Source: CAD feature listing. Evaluate the final solid. Frame: model axes, mm. Coordinates: 2 decimals unless noted, no trailing zeros. Loops run counter-clockwise (first coordinate to the right, second up) from the corner with the lowest first, then second, coordinate; pieces in that order, holes last.
Item 1: Section query C-C, the plane x = 36. Return the cut outline in (y, z).
Item 2: Section query B-B, the plane x = 30. Return the cut outline in (y, z).
Item 3: Pin query (flat end, axial travel): pin 1 Ø1.1 at (y, z) = (-6.5, 0.5) entering from -X (3 decimals); pin 2 Ø1.2 at (x, z) = (11, 0) entering from -Y; pin 3 Ø0.9 at (x, z) = (-12, 0) entering from +Y. Return the tip coordinate at first contact, or that it passes through.
Item 4: Section query A-A, the plane y = 0. Return the cut outline in (x, z) (3 decimals), then the cut area to 3 significant figures.
Item 5: Section query D-D, the plane x = 18. Return the cut outline in (y, z), then the cut area to 3 significant figures.
Item 6: Line query: probe 1 along Y at (x, z) = (30, -0.65); probe 2 along X at (y, z) = (0.5, -0.7) (3 decimals); probe 3 along X at (y, z) = (9, -1.1). Output: solid intervals per line, ascending.
```python
from build123d import *

# Parameters (mm, degrees)
EXTRUDE_1_DEPTH     = 1.25
SKETCH_2_R          = 0.6
CUT_EXTRUDE_1_DEPTH = 3.5
FILLET_1_R          = 0.5
SKETCH_3_R          = 10.5
CUT_EXTRUDE_2_DEPTH = 3.5
CHAMFER_1_SIZE      = 5
CHAMFER_2_SIZE      = 15
CHAMFER_3_SIZE      = 3
CUT_EXTRUDE_4_DEPTH = 3.5
SKETCH_6_R          = 1.55
CUT_EXTRUDE_5_DEPTH = 3.5


with BuildPart() as part:
    # 草图1 → 凸台-拉伸1 (new body, symmetric)
    with BuildSketch(Plane.XY):
        Polygon((-13, 20), (-13, 7.475), (-10.025, 7.475), (-10.025, 4), (-13.025, 4), (-13.025, -4), (-10.025, -4), (-10.025, -7.475), (-13, -7.475), (-13, -30), (42.5, -30), (42.5, 20), align=None)
        Polygon((10.025, 7.475), (10.025, 4), (13.025, 4), (13.025, -4), (10.025, -4), (10.025, -7.475), (16.125, -7.475), (16.125, 7.475), align=None, mode=Mode.SUBTRACT)
    extrude(amount=EXTRUDE_1_DEPTH, both=True)

    # 草图2 → 切除-拉伸1 (cut, through all)
    with BuildSketch(Plane.XY.offset(1.25)):
        with Locations((10.625, 7.475)):
            Circle(SKETCH_2_R)
        with Locations((16.125, 6.875)):
            Circle(SKETCH_2_R)
        with Locations((10.025, 4.6)):
            Circle(SKETCH_2_R)
        with Locations((10.025, -4.6)):
            Circle(SKETCH_2_R)
        with Locations((10.625, -7.475)):
            Circle(SKETCH_2_R)
        with Locations((16.125, -6.875)):
            Circle(SKETCH_2_R)
        with Locations((-10.025, -4.6)):
            Circle(SKETCH_2_R)
        with Locations((-10.625, -7.475)):
            Circle(SKETCH_2_R)
        with Locations((-10.625, 7.475)):
            Circle(SKETCH_2_R)
        with Locations((-10.025, 4.6)):
            Circle(SKETCH_2_R)
    extrude(amount=-CUT_EXTRUDE_1_DEPTH, mode=Mode.SUBTRACT)

    # 圆角1
    fillet_1_edges = [part.edges().sort_by_distance(p)[0] for p in [
        (-13.025, -4, 0),
        (-13.025, 4, 0),
        (13.025, -4, 0),
        (13.025, 4, 0),
    ]]
    fillet(fillet_1_edges, radius=FILLET_1_R)

    # 草图3 → 切除-拉伸2 (cut, through all)
    with BuildSketch(Plane.XY.offset(1.25)):
        with Locations((30, 0)):
            Circle(SKETCH_3_R)
    extrude(amount=-CUT_EXTRUDE_2_DEPTH, mode=Mode.SUBTRACT)

    # 倒角1
    chamfer_1_edges = [part.edges().sort_by_distance(p)[0] for p in [
        (42.5, 20, 0),
    ]]
    chamfer(chamfer_1_edges, length=CHAMFER_1_SIZE)

    # 倒角2
    chamfer_2_edges = [part.edges().sort_by_distance(p)[0] for p in [
        (42.5, -30, 0),
    ]]
    chamfer(chamfer_2_edges, length=CHAMFER_2_SIZE)

    # 倒角3
    chamfer_3_edges = [part.edges().sort_by_distance(p)[0] for p in [
        (-13, -30, 0),
        (-13, 20, 0),
    ]]
    chamfer(chamfer_3_edges, length=CHAMFER_3_SIZE)

    # 草图5 → 切除-拉伸4 (cut, through all)
    with BuildSketch(Plane(origin=(0, 0, -1.25), x_dir=(-1, 0, 0), z_dir=(0, 0, -1))):
        Polygon((-37.5, -20), (-20, -20), (-10, -30), (-27.5, -30), align=None)
    extrude(amount=-CUT_EXTRUDE_4_DEPTH, mode=Mode.SUBTRACT)

    # 草图6 → 切除-拉伸5 (cut, through all)
    with BuildSketch(Plane(origin=(0, 0, -1.25), x_dir=(-1, 0, 0), z_dir=(0, 0, -1))):
        with Locations((-39.545941546, 9.545941546)):
            Circle(SKETCH_6_R)
    extrude(amount=-CUT_EXTRUDE_5_DEPTH, mode=Mode.SUBTRACT)


solid = part.part
```
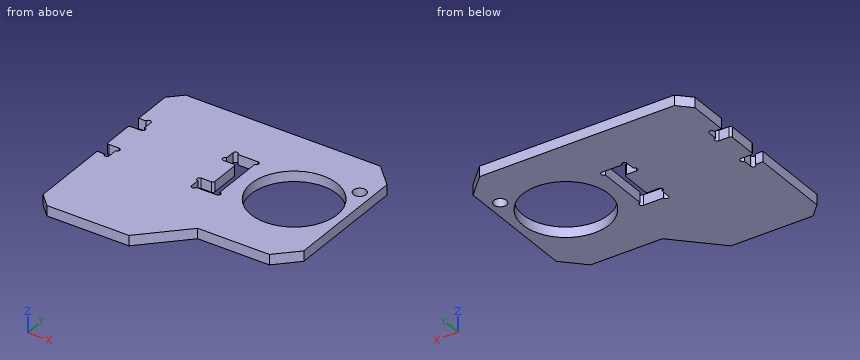
Verdict:
1. outline: (-20, -1.25) - (-8.62, -1.25) - (-8.62, 1.25) - (-20, 1.25) - close; (8.62, -1.25) - (20, -1.25) - (20, 1.25) - (8.62, 1.25) - close
2. outline: (-20, -1.25) - (-10.5, -1.25) - (-10.5, 1.25) - (-20, 1.25) - close; (10.5, -1.25) - (20, -1.25) - (20, 1.25) - (10.5, 1.25) - close
3. pin 1: stops at x = -10.025
3. pin 2: stops at y = -29.6
3. pin 3: stops at y = 18.45
4. outline: (-13.025, -1.25) - (13.025, -1.25) - (13.025, 1.25) - (-13.025, 1.25) - close; (16.125, -1.25) - (19.5, -1.25) - (19.5, 1.25) - (16.125, 1.25) - close; (40.5, -1.25) - (42.5, -1.25) - (42.5, 1.25) - (40.5, 1.25) - close
4. area: 78.6 mm2
5. outline: (-22, -1.25) - (20, -1.25) - (20, 1.25) - (-22, 1.25) - close
5. area: 105 mm2
6. probe 1: y = -20 to -10.5, 10.5 to 20
6. probe 2: x = -13.025 to 13.025, 16.125 to 19.512, 40.488 to 42.5
6. probe 3: x = -13 to 24.59, 35.41 to 38.1, 41 to 42.5
